Check sheet for the modelled part. Datum: model origin and axes. Units: mm. Face numbers are marked on the shaded views. A direction names the side the tool comes from. Give positions to 0.01 mm unless a question says otherwise; leave off trailing zeros. Write each loop counter-clockwise with the first axis right and the second up, starting at its lowest first coordinate (ties: lowest second). Pieces come first, ordered by that corner, then holes. Notation, with made-up numbers: M -5.5,52 L 31.5,52 A23 cw 31.5,62 Z; hole C 53.25,10.5 d4. An arc over 180 degrees is marked long. Use CSV: the item, a comma, the result in double quotes. Start each with the question number.
1. Cross-section at D-D, the plane x = 118.5. Enter the section's corners in (y, z).
2. Access from +Z, -Z, +X, -X, +Y, -Y to the whole of each face (thin tool, end or side, straight path). Record for the marked faces 1, 2 and 3.
3. Cross-section at A-A, the plane z = 50. Enter the section's corners in (x, y), and give its area (3 significant figures).
4. Cross-section at C-C, the plane y = -161. Enter the section's corners in (x, z).
5. Cross-section at B-B, the plane x = 18. Enter the section's corners in (y, z), and give its area (3 significant figures).
6. Scan lines: line 1 (Y direction, x = 37, z = 98.5); line 2 (X direction, y = -160, z = 72.5); line 3 (Z direction, x = 58, y = -73). Record each from-to range of solid material in increasing order.
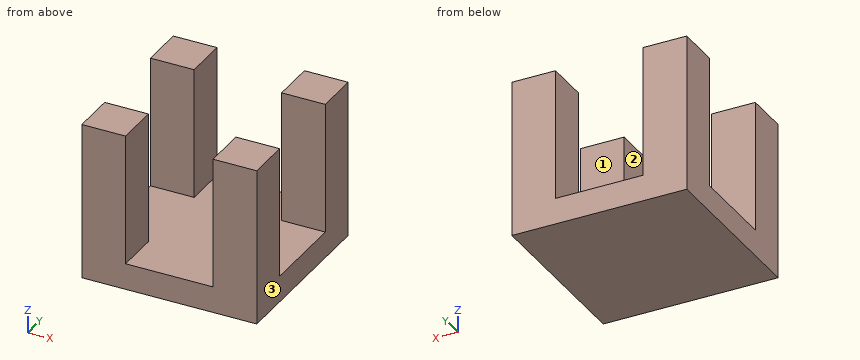
Autodesk Inventor part; units mm, degrees
ref_plane "YZ Plane" through (0, 0, 0) normal (1, 0, 0) x (0, 1, 0)
ref_plane "XZ Plane" through (0, 0, 0) normal (0, 1, 0) x (-1, 0, 0)
ref_plane "XY Plane" through (0, 0, 0) normal (0, 0, 1) x (1, 0, 0)
sketch "Sketch1" plane through (0, 0, 0) normal (0, 0, 1) x (1, 0, 0)
  line L0 (0, 0) -> (0, -200)
  line L1 (0, -200) -> (200, -200)
  line L2 (200, -200) -> (200, 0)
  line L3 (200, 0) -> (0, 0)
  dimension "d0" = 200
  dimension "d1" = 200
extrude "Extrusion1" add sketch "Sketch1" along normal blind 30
sketch "Sketch2" plane through (0, 0, 30) normal (0, 0, 1) x (1, 0, 0)
  line L0 (0, 0) -> (0, -200)
  line L1 (0, 0) -> (0, -50)
  line L2 (0, -50) -> (50, -50)
  line L3 (50, -50) -> (50, 0)
  line L4 (50, 0) -> (0, 0)
  line L5 (200, -200) -> (200, 0)
  line L6 (200, 0) -> (200, -50)
  line L7 (200, -50) -> (150, -50)
  line L8 (150, -50) -> (150, 0)
  line L9 (150, 0) -> (200, 0)
  line L10 (0, -200) -> (0, -150)
  line L11 (0, -150) -> (50, -150)
  line L12 (50, -150) -> (50, -200)
  line L13 (50, -200) -> (0, -200)
  line L14 (200, -200) -> (200, -150)
  line L15 (200, -150) -> (150, -150)
  line L16 (150, -150) -> (150, -200)
  line L17 (150, -200) -> (200, -200)
  dimension "d4" = 50
  dimension "d5" = 50
  dimension "d6" = 50
  dimension "d7" = 50
  dimension "d8" = 50
  dimension "d9" = 50
  dimension "d10" = 50
  dimension "d11" = 50
extrude "Extrusion2" add sketch "Sketch2" along normal blind 150
properties part number "STand_1"
Worked answers:
1,outline,"M -200,0 L 0,0 L 0,30 L -200,30 Z"
2,face 1,"+Z, +X, -X"
2,face 2,"+Z, +Y, -Y"
2,face 3,"+Z, -Z, +X, +Y, -Y"
3,outline,"M 0,-200 L 50,-200 L 50,-150 L 0,-150 Z; M 0,-50 L 50,-50 L 50,0 L 0,0 Z; M 150,-200 L 200,-200 L 200,-150 L 150,-150 Z; M 150,-50 L 200,-50 L 200,0 L 150,0 Z"
3,area,"10,000 mm^2"
4,outline,"M 0,0 L 200,0 L 200,180 L 150,180 L 150,30 L 50,30 L 50,180 L 0,180 Z"
5,outline,"M -200,0 L 0,0 L 0,180 L -50,180 L -50,30 L -150,30 L -150,180 L -200,180 Z"
5,area,"21,000 mm^2"
6,line 1,"y = -200 to -150, -50 to 0"
6,line 2,"x = 0 to 50, 150 to 200"
6,line 3,"z = 0 to 30"
